```python
from build123d import *

# Parameters (mm, degrees)
SKETCH1_R           = 1.6
BOSS_EXTRUDE1_DEPTH = 10
SKETCH2_R           = 1.6
CUT_EXTRUDE1_DEPTH  = 10
SKETCH3_R           = 1.6
BOSS_EXTRUDE2_DEPTH = 10


with BuildPart() as part:
    # Sketch1 → Boss-Extrude1 (new body)
    with BuildSketch(Plane.XY):
        with BuildLine():
            Line((0, 6), (196, 6))
            ThreePointArc((196, 6), (202, 0), (196, -6))
            Line((196, -6), (0, -6))
            ThreePointArc((0, -6), (-6, 0), (0, 6))
        make_face()
        Circle(SKETCH1_R, mode=Mode.SUBTRACT)
        with Locations((196, 0)):
            Circle(SKETCH1_R, mode=Mode.SUBTRACT)
    extrude(amount=BOSS_EXTRUDE1_DEPTH)

    # Sketch2 → Cut-Extrude1 (cut)
    with BuildSketch(Plane.XY.offset(10)):
        with Locations((192, 0)):
            Circle(SKETCH2_R)
        with BuildLine():
            Line((196, 6), (192, 6))
            ThreePointArc((192, 6), (198, 0), (192, -6))
            Line((192, -6), (196, -6))
            ThreePointArc((196, -6), (202, 0), (196, 6))
        make_face()
    extrude(amount=-CUT_EXTRUDE1_DEPTH, mode=Mode.SUBTRACT)

    # Sketch3 → Boss-Extrude2 (add)
    with BuildSketch(Plane.XY.offset(10)):
        with Locations((196, 0)):
            Circle(SKETCH3_R)
    extrude(amount=-BOSS_EXTRUDE2_DEPTH)


solid = part.part
```
Source: CAD feature listing. Evaluate the final solid. Frame: model axes, mm. Give positions to 0.01 mm unless a question says otherwise; leave off trailing zeros. Write each loop counter-clockwise with the first axis right and the second up, starting at its lowest first coordinate (ties: lowest second). Pieces come first, ordered by that corner, then holes.
1. Material intervals for line 1 along Y through (x, z) = (192, 3); line 2 along X through (y, z) = (3.5, 3.5); line 3 along X through (y, z) = (-3, 2.5), sorted ascending.
2. First-contact query: pin 1 (1.5 mm diameter, centred on y = 4, z = 7, fed in from +X); pin 2 (5 mm diameter, centred on y = -3, z = 3, fed in from +X). Flat tips, straight axial feed; report the tip coordinate or a pass-through.
3. Section query A-A (z = 6.5). Return the cut outline in (x, y).
4. Pull-direction query (Y, two-part tool) for faces 1 (the face through (97, 0, 0)), 2 (the face through (95, 6, 5)), 3 (the face through (193.48, -0.61, 5.07)); classes: +Y half, -Y half, draft (parallel to the pull), parting line (faces both ways), or undercut.
Output values:
1. line 1: y = -6 to -1.6, 1.6 to 6
1. line 2: x = -4.87 to 196.87
1. line 3: x = -5.2 to 197.2
2. pin 1: stops at x = 197.04
2. pin 2: stops at x = 197.98
3. outline: (0, -6) - (192, -6) arc R6 ccw to (192, 6) - (0, 6) arc R6 ccw to start; hole circle Ø3.2 at (0, 0); hole circle Ø3.2 at (192, 0)
4. face 1: draft
4. face 2: +Y half
4. face 3: undercut
